```python
from build123d import *

# Parameters (mm, degrees)
SKETCH1_W                  = 107.95
SKETCH1_H                  = 190.5
BOSS_EXTRUDE1_DEPTH        = 12.7
CUT_EXTRUDE1_START         = 12.7
SKETCH2_R                  = 4.7625
CUT_EXTRUDE1_DEPTH         = 3.9624
CUT_EXTRUDE2_START         = -12.7
SKETCH3_R                  = 4.7625
CUT_EXTRUDE2_DEPTH         = 14.6812
SKETCH5_R                  = 4.7625
CUT_EXTRUDE3_DEPTH         = 22.4376
SCALE1_SCALE               = 0.75
SKETCH6_R                  = 2.1336
CUT_EXTRUDE4_DEPTH         = 2.9718
F_10_CLEARANCE_HOLE1_D     = 5.1054
F_10_CLEARANCE_HOLE1_DEPTH = 19.05
FILLET1_R                  = 6.35


with BuildPart() as part:
    # Sketch1 → Boss-Extrude1 (new body, symmetric)
    with BuildSketch(Plane(origin=(0, 0, 0), x_dir=(1, 0, 0), z_dir=(0, 1, 0))):
        with Locations((0, 49.1998)):
            Rectangle(SKETCH1_W, SKETCH1_H)
    extrude(amount=BOSS_EXTRUDE1_DEPTH, both=True)

    # Sketch2 → Cut-Extrude1 (cut)
    with BuildSketch(Plane(origin=(0, 0, 0), x_dir=(1, 0, 0), z_dir=(0, 1, 0)).offset(CUT_EXTRUDE1_START)):
        with BuildLine():
            Line((5.057939535, -14.433014335), (1.190625, 0))
            Line((1.190625, 0), (5.880526895, 0))
            ThreePointArc((5.880526895, 0), (9.472629344, 1.487897552), (10.960526895, 5.08))
            Line((10.960526895, 5.08), (10.960526895, 17.9832))
            ThreePointArc((10.960526895, 17.9832), (9.213211561, 20.396341318), (6.375289871, 19.48938907))
            ThreePointArc((6.375289871, 19.48938907), (6.062916501, 19.358283139), (5.799480669, 19.571279501))
            ThreePointArc((5.799480669, 19.571279501), (4.636397175, 21.079630515), (2.8194, 21.650951144))
            Line((2.8194, 21.650951144), (2.286, 21.650951144))
            ThreePointArc((2.286, 21.650951144), (1.687422653, 22.073983788), (1.886381552, 22.779438829))
            Line((1.886381552, 22.779438829), (21.285138362, 38.488242359))
            ThreePointArc((21.285138362, 38.488242359), (14.964772935, 38.778011994), (14.509654717, 45.088626306))
            Line((14.509654717, 45.088626306), (0, 26.179276127))
            Line((0, 26.179276127), (0, -13.507771027))
            ThreePointArc((0, -13.507771027), (2.570935021, -13.740985226), (5.057939535, -14.433014335))
        make_face()
        with BuildLine():
            Line((3.543726895, 3.048), (2.2225, 3.048))
            Line((2.2225, 3.048), (4.114068772, 8.245042489))
            ThreePointArc((4.114068772, 8.245042489), (4.191366172, 8.399928267), (4.301626576, 8.533371646))
            ThreePointArc((4.301626576, 8.533371646), (4.877320207, 9.368949404), (5.08, 10.3632))
            Line((5.08, 10.3632), (5.08, 16.267431628))
            ThreePointArc((5.08, 16.267431628), (5.809057387, 17.017360952), (6.778491601, 17.40993702))
            ThreePointArc((6.778491601, 17.40993702), (7.090210384, 17.327130128), (7.226726895, 17.034916467))
            Line((7.226726895, 17.034916467), (7.226726895, 6.731))
            ThreePointArc((7.226726895, 6.731), (6.14800117, 4.126725725), (3.543726895, 3.048))
        make_face(mode=Mode.SUBTRACT)
        with Locations((18.288, 42.1894)):
            Circle(SKETCH2_R)
        with BuildLine():
            ThreePointArc((14.2875, -27.795271027), (11.755806382, -19.67531582), (5.057939535, -14.433014335))
            ThreePointArc((5.057939535, -14.433014335), (2.570935021, -13.740985226), (0, -13.507771027))
            Line((0, -13.507771027), (0, -42.082771027))
            ThreePointArc((0, -42.082771027), (10.102788136, -37.898059163), (14.2875, -27.795271027))
        make_face()
    cut_extrude1 = extrude(amount=-CUT_EXTRUDE1_DEPTH, mode=Mode.SUBTRACT)

    # Sketch3 → Cut-Extrude2 (cut)
    with BuildSketch(Plane(origin=(0, 0, 0), x_dir=(1, 0, 0), z_dir=(0, 1, 0)).offset(CUT_EXTRUDE2_START)):
        with BuildLine():
            Line((12.5222, -2.214016109), (4.623727363, 34.945376076))
            ThreePointArc((4.623727363, 34.945376076), (4.751363404, 35.477018448), (5.24485109, 35.7124))
            Line((5.24485109, 35.7124), (14.342303959, 35.7124))
            ThreePointArc((14.342303959, 35.7124), (18.391335215, 36.554087605), (21.769496507, 38.939694118))
            ThreePointArc((21.769496507, 38.939694118), (14.767691653, 38.981778546), (15.375216855, 45.957304006))
            ThreePointArc((15.375216855, 45.957304006), (11.098329565, 43.715563082), (6.311655978, 43.079227305))
            ThreePointArc((6.311655978, 43.079227305), (5.570694317, 43.539610738), (5.580103416, 44.4119))
            Line((5.580103416, 44.4119), (45.923522628, 114.288751826))
            ThreePointArc((45.923522628, 114.288751826), (40.292251924, 132.148860722), (22.990903716, 124.982407647))
            Line((22.990903716, 124.982407647), (0, 61.815418834))
            Line((0, 61.815418834), (0, 1.6764))
            ThreePointArc((0, 1.6764), (6.556310516, 0.681394963), (12.5222, -2.214016109))
        make_face()
        with Locations((18.288, 42.1894)):
            Circle(SKETCH3_R)
        with BuildLine():
            ThreePointArc((22.098, -20.4216), (19.558082467, -10.135540784), (12.5222, -2.214016109))
            ThreePointArc((12.5222, -2.214016109), (6.556310516, 0.681394963), (0, 1.6764))
            Line((0, 1.6764), (0, -42.5196))
            ThreePointArc((0, -42.5196), (15.625645651, -36.047245651), (22.098, -20.4216))
        make_face()
    cut_extrude2 = extrude(amount=CUT_EXTRUDE2_DEPTH, mode=Mode.SUBTRACT)

    # Sketch5 → Cut-Extrude3 (cut, through all)
    with BuildSketch(Plane(origin=(0, 8.7376, 0), x_dir=(1, 0, 0), z_dir=(0, 1, 0))):
        with Locations((18.288, 42.1894)):
            Circle(SKETCH5_R)
    cut_extrude3 = extrude(amount=-CUT_EXTRUDE3_DEPTH, mode=Mode.SUBTRACT)

    # Mirror1: Cut-Extrude1, Cut-Extrude2, Cut-Extrude3 across plane
    add(cut_extrude1.mirror(Plane(origin=(0, 0, 0), x_dir=(0, 0, 1), z_dir=(1, 0, 0))), mode=Mode.SUBTRACT)
    add(cut_extrude2.mirror(Plane(origin=(0, 0, 0), x_dir=(0, 0, 1), z_dir=(1, 0, 0))), mode=Mode.SUBTRACT)
    add(cut_extrude3.mirror(Plane(origin=(0, 0, 0), x_dir=(0, 0, 1), z_dir=(1, 0, 0))), mode=Mode.SUBTRACT)


with BuildPart() as part_1:
    # Scale1: scaled about (0, 0.932530252, -48.998072256)
    add(part.part.scale(SCALE1_SCALE).moved(Location((0, 0.233132563, -12.249518064))))

    # Sketch6 → Cut-Extrude4 (cut)
    with BuildSketch(Plane(origin=(0, 9.758132563, 0), x_dir=(1, 0, 0), z_dir=(0, 1, 0))):
        with Locations((-6.820220171, 20.898218064)):
            Circle(SKETCH6_R)
        with Locations((6.820220171, 20.898218064)):
            Circle(SKETCH6_R)
    extrude(amount=-CUT_EXTRUDE4_DEPTH, mode=Mode.SUBTRACT)

    # #10 Clearance Hole1
    with Locations(Plane(origin=(0, 9.758132563, 0), x_dir=(1, 0, 0), z_dir=(0, 1, 0))):
        with Locations((0, 114.236868064), (-25.4, 53.911868064), (25.4, 53.911868064), (25.4, -9.588131936), (-25.4, -9.588131936)):
            Hole(F_10_CLEARANCE_HOLE1_D / 2, depth=F_10_CLEARANCE_HOLE1_DEPTH)

    # Fillet1
    fillet1_edges = [part_1.edges().sort_by_distance(p)[0] for p in [
        (-40.48125, 0.233132563, -120.586868064),
        (40.48125, 0.233132563, -120.586868064),
        (40.48125, 0.233132563, 22.288131936),
        (-40.48125, 0.233132563, 22.288131936),
    ]]
    fillet(fillet1_edges, radius=FILLET1_R)


solid = part_1.part
```
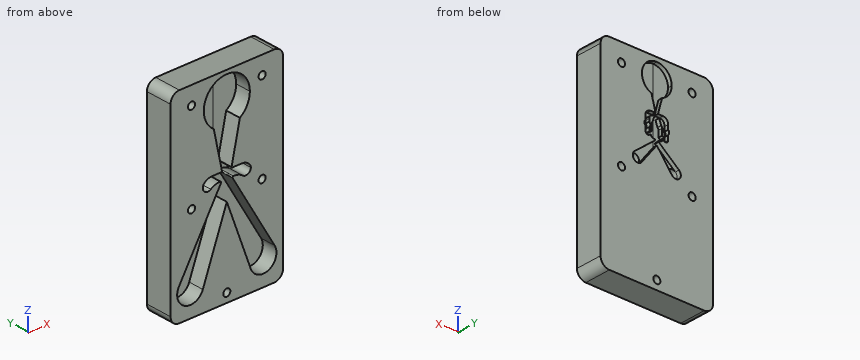
Here's how the part is built. I have some questions about the finished solid (model axes, mm). Give positions to 0.01 mm unless a question says otherwise; leave off trailing zeros. Loops run counter-clockwise (first coordinate to the right, second up) from the corner with the lowest first, then second, coordinate; pieces in that order, holes last. Notation, with made-up numbers: (39.25, 20.25) -> (98.25, 20.25) arc R27 ccw to (98.25, 49.25) -> close; hole circle Ø7 at (-3, 50.25). An arc over 180 degrees is marked (long way). Use one line per item in the form item = value. Start each with the question number.
1) Imagine slicing it at B-B (y = 5.25). Please give me the cut outline in (x, z).
2) Please list where these lines run through material, in increasing order: line 1 along Z through (x, y) = (25.4, 5); line 2 along X through (y, z) = (-3.25, -84); line 3 along Z through (x, y) = (-25, 2.5).
3) Imagine slicing it at D-D (z = -4). Please give me the cut outline in (x, y), then the cut area to 3 significant figures.
4) Imagine slicing it at A-A (x = 14). Please give me the cut outline in (y, z).
5) Imagine slicing it at C-C (x = -25.4). Please give me the cut outline in (y, z).
6) For P1, Ø11.5, axis at x = -13.72, z = -43.89, coming from the -Y side; P2, Ø0.8, axis at x = 7.5, z = -21.5, coming from the +Y side; P3, Ø11.5, axis at x = 26.19, z = -102.73, coming from the -Y side, each with a flat end and sliding along its axis, tell me the tip position at first contact or that it passes through.
Check values:
q1.outline = (-40.48, -114.24) arc R6.35 ccw to (-34.13, -120.59) -> (34.13, -120.59) arc R6.35 ccw to (40.48, -114.24) -> (40.48, 15.94) arc R6.35 ccw to (34.13, 22.29) -> (-34.13, 22.29) arc R6.35 ccw to (-40.48, 15.94) -> close; hole circle Ø5.11 at (-25.4, -53.91); hole circle Ø5.11 at (-25.4, 9.59); hole circle Ø7.14 at (-13.72, -43.89); hole circle Ø5.11 at (0, -114.24); hole circle Ø7.14 at (13.72, -43.89); hole circle Ø5.11 at (25.4, -53.91); hole circle Ø5.11 at (25.4, 9.59)
q2.line_1 = -120.59 to -56.46, -51.36 to 7.04, 12.14 to 22.29
q2.line_2 = -40.48 to -26.38, -9.24 to 9.24, 26.38 to 40.48
q2.line_3 = -120.59 to -56.43, -51.39 to 7.07, 12.11 to 22.29
q3.outline = (-40.48, -9.29) -> (-14.99, -9.29) -> (-14.99, 1.72) -> (14.99, 1.72) -> (14.99, -9.29) -> (40.48, -9.29) -> (40.48, 9.76) -> (3.1, 9.76) -> (3.1, 6.79) -> (-3.1, 6.79) -> (-3.1, 9.76) -> (-40.48, 9.76) -> close
q3.area = 1,190 mm^2
q4.outline = (-9.29, -120.59) -> (9.76, -120.59) -> (9.76, -47.45) -> (-9.29, -47.45) -> (-9.29, -62.56) -> (1.72, -62.56) -> (1.72, -97.08) -> (-9.29, -97.08) -> close; (-9.29, -39.76) -> (1.72, -39.76) -> (1.72, -40.33) -> (6.79, -40.33) -> (6.79, -39.53) -> (9.76, -39.53) -> (9.76, 22.29) -> (-9.29, 22.29) -> (-9.29, 11.94) -> (1.72, 11.94) -> (1.72, -5.8) -> (-9.29, -5.8) -> close
q5.outline = (-9.29, -120.59) -> (9.76, -120.59) -> (9.76, -56.46) -> (-9.29, -56.46) -> (-9.29, -82.3) -> (1.72, -82.3) -> (1.72, -112.22) -> (-9.29, -112.22) -> close; (-9.29, -51.36) -> (9.76, -51.36) -> (9.76, 7.04) -> (-9.29, 7.04) -> close; (-9.29, 12.14) -> (9.76, 12.14) -> (9.76, 22.29) -> (-9.29, 22.29) -> close
q6.P1 = -9.29
q6.P2 = 6.79
q6.P3 = 1.72
